Source: CAD feature listing. Evaluate the final solid. Frame: model axes, mm. Face numbers are marked on the shaded views. Coordinates: 2 decimals unless noted, no trailing zeros. Order: outer loops, then holes, each group sorted by start corner. A loop starts at its lowest first (then second) coordinate and runs counter-clockwise, first axis right, second up.
Item 1: Ray query, line 1 (Y direction, x = 167, z = 186); line 2 (X direction, y = 1, z = 89); line 3 (X direction, y = 3.5, z = 73). Return the intervals inside material, ascending.
Item 2: Mould query, pull axis X, two halves, no side actions, for the marked faces 1 and 2. Classes: released by +X, released by -X, zero draft, split by the parting line, or undercut.
Item 3: Contact query for flat-ended pins moving along their axis: P1, Ø8, axis at y = 9.5, z = 213, coming from the +X side; P2, Ø4, axis at y = 4, z = 51.5, coming from the -X side; P3, Ø8, axis at y = 3, z = 120.5, coming from the +X side. Output: stop coordinate, or through.
Item 4: Section A-A on y = 8.75. Return the cut outline in (x, z), then the cut area to 3 significant figures.
Item 5: Section C-C on x = 253. Return the cut outline in (y, z).
Item 6: Section B-B on z = 105.5. Return the cut outline in (x, y).
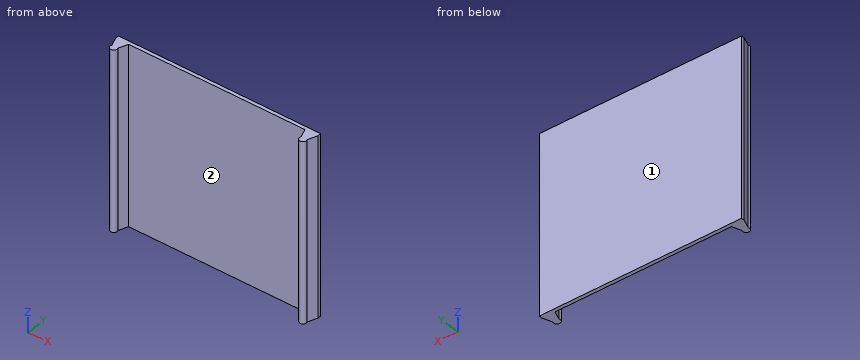
from build123d import *

# Parameters (mm, degrees)
BOSS_EXTRUDE1_DEPTH = 254


with BuildPart() as part:
    # Sketch1 → Boss-Extrude1 (new body)
    with BuildSketch(Plane.XY):
        with BuildLine():
            Line((-9.095097891, 15), (-4.363484846, 2))
            ThreePointArc((-4.363484846, 2), (0, -4.8), (4.363484846, 2))
            Line((4.363484846, 2), (9.095097891, 15))
            Line((9.095097891, 15), (260.044118109, 15))
            Line((260.044118109, 15), (264.775731154, 2))
            ThreePointArc((264.775731154, 2), (269.139216, -4.8), (273.502700846, 2))
            Line((273.502700846, 2), (278.234313891, 15))
            Line((278.234313891, 15), (278.234313891, 20))
            Line((278.234313891, 20), (-9.095097891, 20))
            Line((-9.095097891, 20), (-9.095097891, 15))
        make_face()
    extrude(amount=BOSS_EXTRUDE1_DEPTH)


solid = part.part
Answer list:
1. line 1: y = 15 to 20
1. line 2: x = -4.69 to 4.69, 264.44 to 273.83
1. line 3: x = -4.91 to 4.91, 264.23 to 274.05
2. face 1: zero draft
2. face 2: undercut
3. P1: stops at x = 277.69
3. P2: stops at x = -5.82
3. P3: stops at x = 275.32
4. outline: (-6.82, 0) - (6.82, 0) - (6.82, 254) - (-6.82, 254) - close; (262.32, 0) - (275.96, 0) - (275.96, 254) - (262.32, 254) - close
4. area: 6,930 mm2
5. outline: (15, 0) - (20, 0) - (20, 254) - (15, 254) - close
6. outline: (-9.1, 15) - (-4.36, 2) arc R4.8 ccw (long way) to (4.36, 2) - (9.1, 15) - (260.04, 15) - (264.78, 2) arc R4.8 ccw (long way) to (273.5, 2) - (278.23, 15) - (278.23, 20) - (-9.1, 20) - close
